```python
from build123d import *

# Parameters (mm, degrees)
BOSS_EXTRUDE1_DEPTH    = 3.175
F_10_CLEARANCE_HOLE1_D = 4.9784


with BuildPart() as part:
    # Sketch1 → Boss-Extrude1 (new body)
    with BuildSketch(Plane.XY):
        Polygon((-254.000000508, 0), (-267.103367516, 0), (-267.103367516, 63.5), (-254.000000508, 63.5), (-254.000000508, 25.666043074), (-241.033957434, 12.7), (-203.200000508, 12.7), (-203.200000508, 0), align=None)
    extrude(amount=BOSS_EXTRUDE1_DEPTH)

    # #10 Clearance Hole1 (through all)
    with Locations(Plane.XY.offset(3.175)):
        with Locations((-260.551684012, 6.388229415), (-260.551684012, 25.438229415), (-260.551684012, 50.8), (-241.501684012, 6.388229415), (-216.101684012, 6.388229415)):
            Hole(F_10_CLEARANCE_HOLE1_D / 2)


solid = part.part
```
Model file for the job. Use its own axes, mm. A direction names the side the tool comes from. Round coordinates to 2 decimals unless told otherwise and drop trailing zeros. Write each loop counter-clockwise with the first axis right and the second up, starting at its lowest first coordinate (ties: lowest second). Pieces come first, ordered by that corner, then holes. Notation, with made-up numbers: (84.5, 21) - (97.5, 21) arc R28 ccw to (97.5, 54) - close; hole circle Ø8 at (-7.75, -17.75). An arc over 180 degrees is marked (long way). Use CSV: the item, a comma, the result in double quotes. Start each with the question number.
Item 1: Tool access for faces 1 (the face through (-258.065, 25.548, 1.565)), 2 (the face through (-222, 12.7, 2)): list every direction of +Z, -Z, +X, -X, +Y, -Y with a clear straight run to the whole face (end or side of a thin tool).
Item 2: Band-saw the part on B-B (z = 2.1). Write the cut outline in (x, y), and give its area (3 significant figures).
Item 3: Two-plate mould, pull along X, no slides. Class faces 3 (the face through (-254, 45, 2)), 4 (the face through (-243.876, 7.136, 1.565)), 5 (the face through (-249, 18, 3.175)): released by +X, released by -X, zero draft, split by the parting line, or undercut.
Item 4: Pin check, flat tips, straight feed: P1, Ø12, axis at x = -258, y = 16.5, coming from the -Z side; P2, Ø1.6, axis at y = 36, z = 2, coming from the +X side. Stop position of each tip, or through.
Item 5: Band-saw the part on C-C (x = -223). Write the cut outline in (y, z) (3 decimals).
Item 6: Drill centre lines: L1, parallel to X at y = 50.5, z = 1.1; L2, parallel to Y at x = -206, z = 1.45; L3, parallel to X at y = 6, z = 3. Where is each one in solid material? Low to high. Write a range as [from, to].
Item 7: Band-saw the part on D-D (y = 39.5). Write the cut outline in (x, z) (3 decimals).
Item 8: Band-saw the part on A-A (y = 50.8). Write the cut outline in (x, z) (3 decimals).
Checked values:
1,face 1,"+Z, -Z"
1,face 2,"+Z, -Z, +X, +Y"
2,outline,"(-267.1, 0) - (-203.2, 0) - (-203.2, 12.7) - (-241.03, 12.7) - (-254, 25.67) - (-254, 63.5) - (-267.1, 63.5) - close; hole circle Ø4.98 at (-260.55, 6.39); hole circle Ø4.98 at (-260.55, 25.44); hole circle Ø4.98 at (-260.55, 50.8); hole circle Ø4.98 at (-241.5, 6.39); hole circle Ø4.98 at (-216.1, 6.39)"
2,area,"1,460 mm²"
3,face 3,"released by +X"
3,face 4,"undercut"
3,face 5,"zero draft"
4,P1,"stops at z = 0"
4,P2,"stops at x = -254"
5,outline,"(0, 0) - (12.7, 0) - (12.7, 3.175) - (0, 3.175) - close"
6,L1,"x = [-267.1, -263.02], [-258.08, -254]"
6,L2,"y = [0, 12.7]"
6,L3,"x = [-267.1, -263.01], [-258.09, -243.96], [-239.04, -218.56], [-213.64, -203.2]"
7,outline,"(-267.103, 0) - (-254, 0) - (-254, 3.175) - (-267.103, 3.175) - close"
8,outline,"(-267.103, 0) - (-263.041, 0) - (-263.041, 3.175) - (-267.103, 3.175) - close; (-258.062, 0) - (-254, 0) - (-254, 3.175) - (-258.062, 3.175) - close"
